Input: part model. Units: mm. Frame: model coordinates. Face numbers are marked on the shaded views. A direction names the side the tool comes from. Give positions to 0.01 mm unless a question says otherwise; leave off trailing zeros. Loops run counter-clockwise (first coordinate to the right, second up) from the corner with the lowest first, then second, coordinate; pieces in that order, holes last.
from build123d import *

# Parameters (mm, degrees)
CYLINDER095_R     = 10
CYLINDER095_DEPTH = 34
CYLINDER093_R     = 1.5
CYLINDER093_DEPTH = 14
CYLINDER090_R     = 12.5
CYLINDER090_DEPTH = 33
CYLINDER094_R     = 1.5
CYLINDER094_DEPTH = 14
CYLINDER088_R     = 14
CYLINDER088_DEPTH = 33
BOX016_W          = 1
BOX016_H          = 1
BOX016_DEPTH      = 1
CYLINDER084_R     = 17
CYLINDER084_DEPTH = 5
CYLINDER_R        = 19
CYLINDER_DEPTH    = 34


with BuildPart() as cylinder001:
    # Cylinder095 → Cylinder095 (new body)
    with BuildSketch(Plane.XY.offset(-33)):
        Circle(CYLINDER095_R)
    extrude(amount=CYLINDER095_DEPTH)


with BuildPart() as obj1:
    # Cylinder093 → Cylinder093 (new body)
    with BuildSketch(Plane(origin=(53.66, 148, -15), x_dir=(1, 0, 0), z_dir=(0, 0, 1))):
        Circle(CYLINDER093_R)
    extrude(amount=CYLINDER093_DEPTH)


with BuildPart() as obj2:
    # Cylinder090 → Cylinder090 (new body)
    with BuildSketch(Plane(origin=(73.66, 148, -10), x_dir=(1, 0, 0), z_dir=(0, 0, 1))):
        Circle(CYLINDER090_R)
    extrude(amount=CYLINDER090_DEPTH)


with BuildPart() as fusion039:
    # Cylinder094 → Cylinder094 (new body)
    with BuildSketch(Plane(origin=(93.66, 148, -14), x_dir=(1, 0, 0), z_dir=(0, 0, 1))):
        Circle(CYLINDER094_R)
    extrude(amount=CYLINDER094_DEPTH)

    # Fusion039: union obj1, obj2
    add(obj1.part)
    add(obj2.part)


with BuildPart() as obj3:
    # Cylinder088 → Cylinder088 (new body)
    with BuildSketch(Plane(origin=(73.66, 148, -10), x_dir=(1, 0, 0), z_dir=(0, 0, 1))):
        Circle(CYLINDER088_R)
    extrude(amount=CYLINDER088_DEPTH)


with BuildPart() as obj4:
    # Box016 → Box016 (new body)
    with BuildSketch(Plane(origin=(63, 136, -8), x_dir=(1, 0, 0), z_dir=(0, 0, 1))):
        with Locations((0.5, 0.5)):
            Rectangle(BOX016_W, BOX016_H)
    extrude(amount=BOX016_DEPTH)


with BuildPart() as obj5:
    # Cylinder084 → Cylinder084 (new body)
    with BuildSketch(Plane(origin=(73.66, 148, -10), x_dir=(1, 0, 0), z_dir=(0, 0, 1))):
        Circle(CYLINDER084_R)
    extrude(amount=CYLINDER084_DEPTH)

    # Fusion038: union obj3, obj4
    add(obj3.part)
    add(obj4.part)

    # Cut010: cut Fusion039
    add(fusion039.part, mode=Mode.SUBTRACT)


with BuildPart() as obj5_1:
    # Cut010 placement: moved
    add(obj5.part.moved(Location((-73.66, -148, -23))))


with BuildPart() as cut011:
    # Cylinder → Cylinder (new body)
    with BuildSketch(Plane.XY.offset(-33)):
        Circle(CYLINDER_R)
    extrude(amount=CYLINDER_DEPTH)

    # Cut: cut obj5
    add(obj5_1.part, mode=Mode.SUBTRACT)

    # Cut011: cut Cylinder001
    add(cylinder001.part, mode=Mode.SUBTRACT)


solid = cut011.part
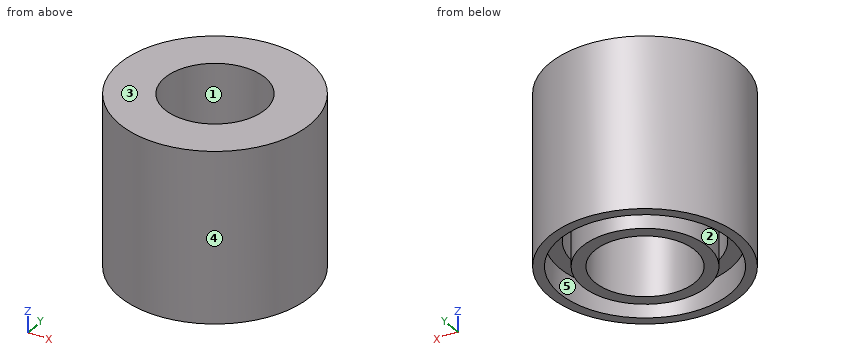
(1) Pin query (flat end, axial travel): pin 1 Ø12 at (y, z) = (-7.5, -22) entering from -X; pin 2 Ø6 at (y, z) = (5, -26.5) entering from +X; pin 3 Ø3 at (y, z) = (8.5, -28) entering from -X. Return the tip coordinate at first contact, or that it passes through.
Values follow:
pin 1: stops at x = -18.94
pin 2: stops at x = 18.89
pin 3: stops at x = -17.66
(2) Cut plane B-B (x = 3). Return the cut outline in (y, z), and give its area (3 significant figures).
Values follow:
outline: (-18.76, -33) - (-16.73, -33) - (-16.73, -28) - (-13.67, -28) - (-13.67, 0) - (-12.13, 0) - (-12.13, -33) - (-9.54, -33) - (-9.54, 1) - (-18.76, 1) - close; (9.54, -33) - (12.13, -33) - (12.13, 0) - (13.67, 0) - (13.67, -28) - (16.73, -28) - (16.73, -33) - (18.76, -33) - (18.76, 1) - (9.54, 1) - close
area: 495 mm2
(3) Ray query, probe 1 along Y at (x, z) = (0, -31.1); probe 2 along Y at (x, z) = (0, -18); probe 3 along X at (y, z) = (5, -6). Return the intervals inside material, ascending.
Values follow:
probe 1: y = -19 to -17, -12.5 to -10, 10 to 12.5, 17 to 19
probe 2: y = -19 to -14, -12.5 to -10, 10 to 12.5, 14 to 19
probe 3: x = -18.33 to -13.08, -11.46 to -8.66, 8.66 to 11.46, 13.08 to 18.33
(4) Cut plane A-A (y = 0). Return the cut outline in (x, z), and give its area (3 significant figures).
Values follow:
outline: (-19, -33) - (-17, -33) - (-17, -28) - (-14, -28) - (-14, 0) - (-12.5, 0) - (-12.5, -33) - (-10, -33) - (-10, 1) - (-19, 1) - close; (10, -33) - (12.5, -33) - (12.5, 0) - (14, 0) - (14, -28) - (17, -28) - (17, -33) - (19, -33) - (19, 1) - (10, 1) - close
area: 483 mm2
(5) Cut plane C-C (z = -24.5). Return the cut outline in (x, y), and give its area (3 significant figures).
Values follow:
outline: circle Ø38 at (0, 0); circle Ø25 at (0, 0); hole circle Ø28 at (0, 0); hole circle Ø20 at (0, 0)
area: 695 mm2
(6) Reachability of the marked faces 1 and 2 from +Z, -Z, +X, -X, +Y, -Y: full face, straight path, thin tool, end or side. Return the list, or none.
Values follow:
face 1: +Z, -Z
face 2: -Z
(7) Mould query, pull axis X, two halves, no side actions, for the marked faces 3, 4 and 5. Classes: +X half, -X half, draft (parallel to the pull), parting line (faces both ways), or undercut.
Values follow:
face 3: draft
face 4: parting line
face 5: undercut
(8) Cut plane D-D (y = 15). Return the cut outline in (x, z), and give its area (3 significant figures).
Values follow:
outline: (-11.66, -33) - (-8, -33) - (-8, -28) - (8, -28) - (8, -33) - (11.66, -33) - (11.66, 1) - (-11.66, 1) - close
area: 713 mm2
